CAD build for the part. Positions are in the model's coordinates, mm. A direction names the side the tool comes from. Coordinates: 2 decimals unless noted, no trailing zeros. Loops run counter-clockwise (first coordinate to the right, second up) from the corner with the lowest first, then second, coordinate; pieces in that order, holes last. Notation, with made-up numbers: (-15, 25.5) -> (37, 25.5) arc R27 cw to (37, 42.5) -> close; hole circle Ø1 at (0.25, 81). An arc over 180 degrees is marked (long way). Return JSON: item names as keys, results as strings. Group by question number.
(1) Probe L1, parallel to Z at x = -2, y = 43.5; L2, parallel to X at y = 39, z = 1.5; L3, parallel to Z at x = -2, y = 4. List the from-to ranges inside material, lowest first.
(2) Tool access for faces 1 (the face through (0, 38, 25)), 2 (the face through (1, 0, -1)): list every direction of +Z, -Z, +X, -X, +Y, -Y with a clear straight run to the whole face (end or side of a thin tool).
(3) Mould opens along Z. For faces 3 (the face through (1, 50.8, 40)), 4 (the face through (-89.885, 25.044, -19.96)), 5 (the face through (-15, 38, 31.35)) say: pulls with the +Z half, pulls with the -Z half, needs draft (parallel to the pull), parting line crosses it, or undercut.
(4) Saw through at D-D on y = 16.5. Write the cut outline in (x, z) (3 decimals).
(5) Saw through at B-B on x = 0. Write the cut outline in (y, z) (3 decimals), then the cut area to 3 significant figures.
(6) Flat gauge pins, fed straight in: pin 1 Ø6 at (y, z) = (9.5, -30.5) entering from -X; pin 2 Ø1 at (y, z) = (19, -42) entering from -X; pin 3 Ø3.5 at (y, z) = (37, -29.5) entering from +X. Where does each tip first touch, or does it go through?
(7) Saw through at C-C on z = 0. Write the cut outline in (x, y) (3 decimals), then the cut area to 3 significant figures.
```python
from build123d import *

# Parameters (mm, degrees)
SKETCH1_R           = 92.075
BOSS_EXTRUDE1_DEPTH = 50.8
CUT_EXTRUDE1_DEPTH  = 25.4


with BuildPart() as part:
    # Sketch1 → Boss-Extrude1 (new body)
    with BuildSketch(Plane(origin=(0, 0, 0), x_dir=(1, 0, 0), z_dir=(0, 1, 0))):
        with Locations(Location((0, 0, 0), (0, 0, 270))):
            Circle(SKETCH1_R)
    extrude(amount=BOSS_EXTRUDE1_DEPTH)

    # Sketch2 → Cut-Extrude1 (cut)
    with BuildSketch(Plane(origin=(0, 50.8, 0), x_dir=(1, 0, 0), z_dir=(0, 1, 0))):
        with BuildLine():
            Line((-67.611774054, 6.149716593), (-67.611774054, 4.988825845))
            Line((-67.611774054, 4.988825845), (-67.611774054, -4.988825845))
            Line((-67.611774054, -4.988825845), (-67.611774054, -6.149716593))
            ThreePointArc((-67.611774054, -6.149716593), (-67.505615069, -6.598100625), (-67.209677573, -6.95128467))
            Line((-67.209677573, -6.95128467), (-47.801200772, -21.428403847))
            ThreePointArc((-47.801200772, -21.428403847), (-33.655307467, -28.804821632), (-17.906024822, -31.35))
            Line((-17.906024822, -31.35), (-12.5, -31.35))
            Line((-12.5, -31.35), (-12.5, -27))
            ThreePointArc((-12.5, -27), (-11.914213562, -25.585786438), (-10.5, -25))
            Line((-10.5, -25), (-0.667840434, -25))
            Line((-0.667840434, -25), (0.667840434, -25))
            Line((0.667840434, -25), (10.5, -25))
            ThreePointArc((10.5, -25), (11.914213562, -25.585786438), (12.5, -27))
            Line((12.5, -27), (12.5, -31.35))
            Line((12.5, -31.35), (17.906024822, -31.35))
            ThreePointArc((17.906024822, -31.35), (33.655307467, -28.804821632), (47.801200772, -21.428403847))
            Line((47.801200772, -21.428403847), (67.209677573, -6.95128467))
            ThreePointArc((67.209677573, -6.95128467), (67.505615069, -6.598100625), (67.611774054, -6.149716593))
            Line((67.611774054, -6.149716593), (67.611774054, -4.988825845))
            Line((67.611774054, -4.988825845), (67.611774054, 4.988825845))
            Line((67.611774054, 4.988825845), (67.611774054, 6.149716593))
            ThreePointArc((67.611774054, 6.149716593), (67.505615069, 6.598100625), (67.209677573, 6.95128467))
            Line((67.209677573, 6.95128467), (47.801200772, 21.428403847))
            ThreePointArc((47.801200772, 21.428403847), (33.655307467, 28.804821632), (17.906024822, 31.35))
            Line((17.906024822, 31.35), (12.5, 31.35))
            Line((12.5, 31.35), (12.5, 27))
            ThreePointArc((12.5, 27), (11.914213562, 25.585786438), (10.5, 25))
            Line((10.5, 25), (0.667840434, 25))
            Line((0.667840434, 25), (-0.667840434, 25))
            Line((-0.667840434, 25), (-10.5, 25))
            ThreePointArc((-10.5, 25), (-11.914213562, 25.585786438), (-12.5, 27))
            Line((-12.5, 27), (-12.5, 31.35))
            Line((-12.5, 31.35), (-17.906024822, 31.35))
            ThreePointArc((-17.906024822, 31.35), (-33.655307467, 28.804821632), (-47.801200772, 21.428403847))
            Line((-47.801200772, 21.428403847), (-67.209677573, 6.95128467))
            ThreePointArc((-67.209677573, 6.95128467), (-67.505615069, 6.598100625), (-67.611774054, 6.149716593))
        make_face()
    extrude(amount=-CUT_EXTRUDE1_DEPTH, mode=Mode.SUBTRACT)


solid = part.part
```
Geometry results:
{
 "1": {"L1": "-92.05 to -25, 25 to 92.05", "L2": "-92.06 to -67.61, 67.61 to 92.06", "L3": "-92.05 to 92.05"},
 "2": {"face 1": "+Y", "face 2": "+Z, -Z, +X, -X, -Y"},
 "3": {"face 3": "needs draft", "face 4": "parting line crosses it", "face 5": "undercut"},
 "4": {"outline": "circle Ø184.15 at (0, 0)"},
 "5": {"outline": "(0, -92.075) -> (50.8, -92.075) -> (50.8, -25) -> (25.4, -25) -> (25.4, 25) -> (50.8, 25) -> (50.8, 92.075) -> (0, 92.075) -> close", "area": "8,080 mm²"},
 "6": {"pin 1": "x = -87.87", "pin 2": "x = -82.19", "pin 3": "x = 87.79"},
 "7": {"outline": "(-92.075, 0) -> (92.075, 0) -> (92.075, 50.8) -> (67.612, 50.8) -> (67.612, 25.4) -> (-67.612, 25.4) -> (-67.612, 50.8) -> (-92.075, 50.8) -> close", "area": "5,920 mm²"}
}
